Check sheet for the modelled part. Datum: model origin and axes. Units: mm. A direction names the side the tool comes from. Round coordinates to 2 decimals unless told otherwise and drop trailing zeros. Order: outer loops, then holes, each group sorted by start corner. A loop starts at its lowest first (then second) coordinate and runs counter-clockwise, first axis right, second up.
(1) Tool access check on faces 5 (the flat face through (-23, 26.7, 0)), 6 (the cylindrical face through (-13.517, 40.125, -0.759)), 7 (the flat face through (0, 19, 10)), 8 (the flat face through (23, 26.7, 0)), 9 (the flat face through (-23, 29.2, 0)). Record the directions out of +Z, -Z, +X, -X, +Y, -Y that give a thin tool (end or side, any length) a straight path to the whole face; none if there is none.
(2) Sectioned sample at D-D, the plane y = 24. Enter the section's corners in (x, z).
(3) Sectioned sample at A-A, the plane x = -24.1. Enter the section's corners in (y, z), and give its area (3 significant figures).
(4) Mould release check, pull along X, two halves, no side actions. Record for faces 1 (the flat face through (26.7, 28, 8)), 2 (the flat face through (-26.7, 28, -8)), 3 (the cylindrical face through (21.9, 27.9, 4.9)), 4 (the cylindrical face through (21.9, 27.9, -5)): released by +X, released by -X, zero draft, split by the parting line, or undercut.
(5) Sectioned sample at B-B, the plane z = 4.95. Enter the section's corners in (x, y).
(6) Sectioned sample at C-C, the plane x = -10.1. Enter the section's corners in (y, z), and give its area (4 significant figures).
(7) Thickness scan on probe 1 along Z at (x, y) = (-24.1, 27.7); probe 2 along Y at (x, z) = (-8.5, 8.25); probe 3 along Y at (x, z) = (-23, 1.75). Record the ranges inside material, lowest first.
(8) Depth check by flat-ended pin: pin 1 (5 mm diameter, centred on x = 24, z = -2.5, fed in from -Y); pin 2 (1 mm diameter, centred on y = 14, z = -6.5, fed in from +X); pin 3 (7 mm diameter, centred on x = -24.1, z = 4.95, fed in from +Y). Enter the tip coordinate at first touch or a pass-through.
```python
from build123d import *

# Parameters (mm, degrees)
SKETCH1_W           = 40.3
SKETCH1_H           = 20
BOSS_EXTRUDE1_DEPTH = 38.4
BOSS_EXTRUDE3_START = -11.7
BOSS_EXTRUDE3_DEPTH = 2.5
SKETCH5_R           = 3.5
BOSS_EXTRUDE4_DEPTH = 3.5


with BuildPart() as part:
    # Sketch1 → Boss-Extrude1 (new body)
    with BuildSketch(Plane(origin=(0, 0, 0), x_dir=(1, 0, 0), z_dir=(0, 1, 0))):
        Rectangle(SKETCH1_W, SKETCH1_H)
    extrude(amount=BOSS_EXTRUDE1_DEPTH)

    # Sketch3 → Boss-Extrude3 (add)
    with BuildSketch(Plane(origin=(0, 38.4, 0), x_dir=(1, 0, 0), z_dir=(0, 1, 0)).offset(BOSS_EXTRUDE3_START)):
        with BuildLine():
            Line((-26.7, 10), (26.7, 10))
            Line((26.7, 10), (26.7, 6.455172275))
            Line((26.7, 6.455172275), (25.704511273, 6.455172275))
            ThreePointArc((25.704511273, 6.455172275), (21.9, 4.95), (25.704511273, 3.444827725))
            Line((25.704511273, 3.444827725), (26.7, 3.444827725))
            Line((26.7, 3.444827725), (26.7, -3.444827725))
            Line((26.7, -3.444827725), (25.704511273, -3.444827725))
            ThreePointArc((25.704511273, -3.444827725), (21.9, -4.95), (25.704511273, -6.455172275))
            Line((25.704511273, -6.455172275), (26.7, -6.455172275))
            Line((26.7, -6.455172275), (26.7, -10))
            Line((26.7, -10), (-26.7, -10))
            Line((-26.7, -10), (-26.7, -6.455172275))
            Line((-26.7, -6.455172275), (-25.704511273, -6.455172275))
            ThreePointArc((-25.704511273, -6.455172275), (-21.9, -4.95), (-25.704511273, -3.444827725))
            Line((-25.704511273, -3.444827725), (-26.7, -3.444827725))
            Line((-26.7, -3.444827725), (-26.7, 3.444827725))
            Line((-26.7, 3.444827725), (-25.704511273, 3.444827725))
            ThreePointArc((-25.704511273, 3.444827725), (-21.9, 4.95), (-25.704511273, 6.455172275))
            Line((-25.704511273, 6.455172275), (-26.7, 6.455172275))
            Line((-26.7, 6.455172275), (-26.7, 10))
        make_face()
    extrude(amount=BOSS_EXTRUDE3_DEPTH)

    # Sketch5 → Boss-Extrude4 (add)
    with BuildSketch(Plane(origin=(0, 38.4, 0), x_dir=(1, 0, 0), z_dir=(0, 1, 0))):
        with Locations(Location((-10.1, 0, 0), (0, 0, 270))):
            Circle(SKETCH5_R)
    extrude(amount=BOSS_EXTRUDE4_DEPTH)


solid = part.part
```
Derived:
1. face 5: +Z, -Z, -X, -Y
1. face 6: +Y
1. face 7: +Z, +X, -X, +Y, -Y
1. face 8: +Z, -Z, +X, -Y
1. face 9: +Z, -Z, -X, +Y
2. outline: (-20.15, -10) - (20.15, -10) - (20.15, 10) - (-20.15, 10) - close
3. outline: (26.7, -10) - (29.2, -10) - (29.2, -7.15) - (26.7, -7.15) - close; (26.7, -2.75) - (29.2, -2.75) - (29.2, 2.75) - (26.7, 2.75) - close; (26.7, 7.15) - (29.2, 7.15) - (29.2, 10) - (26.7, 10) - close
3. area: 28.0 mm2
4. face 1: released by +X
4. face 2: released by -X
4. face 3: undercut
4. face 4: undercut
5. outline: (-21.9, 26.7) - (-20.15, 26.7) - (-20.15, 0) - (20.15, 0) - (20.15, 26.7) - (21.9, 26.7) - (21.9, 29.2) - (20.15, 29.2) - (20.15, 38.4) - (-20.15, 38.4) - (-20.15, 29.2) - (-21.9, 29.2) - close
6. outline: (0, -10) - (38.4, -10) - (38.4, -3.5) - (41.9, -3.5) - (41.9, 3.5) - (38.4, 3.5) - (38.4, 10) - (0, 10) - close
6. area: 792.5 mm2
7. probe 1: z = -10 to -7.15, -2.75 to 2.75, 7.15 to 10
7. probe 2: y = 0 to 38.4
7. probe 3: y = 26.7 to 29.2
8. pin 1: stops at y = 26.7
8. pin 2: stops at x = 20.15
8. pin 3: stops at y = 29.2
